Read the model definition and answer for the solid it produces. Units are mm, in the model's axes. Face numbers are marked on the shaded views. A direction names the side the tool comes from. Give positions to 0.01 mm unless a question says otherwise; leave off trailing zeros. Loops run counter-clockwise (first coordinate to the right, second up) from the corner with the lowest first, then second, coordinate; pieces in that order, holes last.
(1) Find section A-A, the plane z = 2. Write down the section's boundary in (x, y), then the cut area to 3 significant figures.
(2) Straight lines are drawn through the part: probe 1 along Y at (x, z) = (6.75, 2); probe 2 along Y at (x, z) = (14, 9.25); probe 3 along X at (y, z) = (15.75, 10). For each, find the intervals that lie inside material, in ascending order.
(3) Find section B-B, the plane y = 8. Write down the section's boundary in (x, z), then the cut area to 3 significant figures.
(4) Find section D-D, the plane y = 3.25. Write down the section's boundary in (x, z).
(5) Find section C-C, the plane x = 11.5. Write down the section's boundary in (y, z), then the cut area to 3 significant figures.
(6) Which of the six approach directions +Z, -Z, +X, -X, +Y, -Y give full straight-line access (tool end or side, diameter ignored) to the marked faces 1, 2, 3 and 4?
(7) Determine the mould class of the marked faces 5, 6, 7 and 8 for opening direction Y: pulls with the +Y half, pulls with the -Y half, needs draft (parallel to the pull), parting line crosses it, or undercut.
(8) Each of these flat-tipped pins is pushed along its axis until it touches: P1, Ø0.7, axis at y = 7.5, z = 7, coming from the +X side; P2, Ø4, axis at x = 6.5, z = 6, coming from the -Y side; P3, Ø2, axis at y = 4.5, z = 5, coming from the -X side. Where does it stop, or does it pass through?
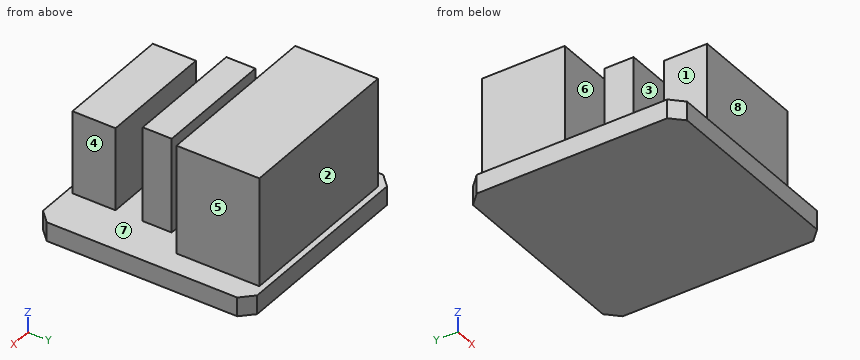
```python
from build123d import *

# Parameters (mm, degrees)
SKETCH1_W           = 18
SKETCH1_H           = 18.1
BOSS_EXTRUDE1_DEPTH = 1.6
CHAMFER1_SIZE       = 1
SKETCH2_W           = 9.9
SKETCH2_H           = 3.64
BOSS_EXTRUDE2_DEPTH = 7
SKETCH3_W           = 10.3
SKETCH3_H           = 2.45
BOSS_EXTRUDE3_DEPTH = 8
SKETCH4_W           = 14.62
SKETCH4_H           = 7
BOSS_EXTRUDE4_DEPTH = 9.2


with BuildPart() as part:
    # Sketch1 → Boss-Extrude1 (new body)
    with BuildSketch(Plane.XY):
        with Locations((9, 9.05)):
            Rectangle(SKETCH1_W, SKETCH1_H)
    extrude(amount=BOSS_EXTRUDE1_DEPTH)

    # Chamfer1
    chamfer1_edges = [part.edges().sort_by_distance(p)[0] for p in [
        (0, 18.1, 0.8),
        (18, 18.1, 0.8),
        (18, 0, 0.8),
        (0, 0, 0.8),
    ]]
    chamfer(chamfer1_edges, length=CHAMFER1_SIZE)

    # Sketch2 → Boss-Extrude2 (add)
    with BuildSketch(Plane.XY.offset(1.6)):
        with Locations((9.15, 2.32)):
            Rectangle(SKETCH2_W, SKETCH2_H)
    extrude(amount=BOSS_EXTRUDE2_DEPTH)

    # Sketch3 → Boss-Extrude3 (add)
    with BuildSketch(Plane.XY.offset(1.6)):
        with Locations((8.95, 7.665)):
            Rectangle(SKETCH3_W, SKETCH3_H)
    extrude(amount=BOSS_EXTRUDE3_DEPTH)

    # Sketch4 → Boss-Extrude4 (add)
    with BuildSketch(Plane.XY.offset(1.6)):
        with Locations((8.69, 14.1)):
            Rectangle(SKETCH4_W, SKETCH4_H)
    extrude(amount=BOSS_EXTRUDE4_DEPTH)


solid = part.part
```
Entries:
1. outline: (1.38, 10.6) - (16, 10.6) - (16, 17.6) - (1.38, 17.6) - close; (3.8, 6.44) - (14.1, 6.44) - (14.1, 8.89) - (3.8, 8.89) - close; (4.2, 0.5) - (14.1, 0.5) - (14.1, 4.14) - (4.2, 4.14) - close
1. area: 164 mm2
2. probe 1: y = 0.5 to 4.14, 6.44 to 8.89, 10.6 to 17.6
2. probe 2: y = 6.44 to 8.89, 10.6 to 17.6
2. probe 3: x = 1.38 to 16
3. outline: (0, 0) - (18, 0) - (18, 1.6) - (14.1, 1.6) - (14.1, 9.6) - (3.8, 9.6) - (3.8, 1.6) - (0, 1.6) - close
3. area: 111 mm2
4. outline: (0, 0) - (18, 0) - (18, 1.6) - (14.1, 1.6) - (14.1, 8.6) - (4.2, 8.6) - (4.2, 1.6) - (0, 1.6) - close
5. outline: (0, 0) - (18.1, 0) - (18.1, 1.6) - (17.6, 1.6) - (17.6, 10.8) - (10.6, 10.8) - (10.6, 1.6) - (8.89, 1.6) - (8.89, 9.6) - (6.44, 9.6) - (6.44, 1.6) - (4.14, 1.6) - (4.14, 8.6) - (0.5, 8.6) - (0.5, 1.6) - (0, 1.6) - close
5. area: 138 mm2
6. face 1: +Z, -X, -Y
6. face 2: +Z, +X, -X, +Y
6. face 3: +Z, +X, -X
6. face 4: +Z, +X, -Y
7. face 5: needs draft
7. face 6: undercut
7. face 7: undercut
7. face 8: pulls with the -Y half
8. P1: stops at x = 14.1
8. P2: stops at y = 0.5
8. P3: stops at x = 4.2
